from build123d import *

# Parameters (mm, degrees)
SKETCH_1_W          = 75
SKETCH_1_H          = 15
EXTRUDE_1_DEPTH     = 2
FILLET_1_R          = 7.5
SKETCH_2_R          = 4.5
SKETCH_2_R_2        = 2
CUT_EXTRUDE_1_DEPTH = 2
CUT_EXTRUDE_3_DEPTH = 10
FILLET_5_R          = 1


with BuildPart() as part:
    # 草图1 → 凸台-拉伸1 (new body)
    with BuildSketch(Plane.XY):
        Rectangle(SKETCH_1_W, SKETCH_1_H)
    extrude(amount=EXTRUDE_1_DEPTH)

    # 圆角1
    fillet_1_edges = [part.edges().sort_by_distance(p)[0] for p in [
        (37.5, -7.5, 1),
        (-37.5, -7.5, 1),
        (-37.5, 7.5, 1),
        (37.5, 7.5, 1),
    ]]
    fillet(fillet_1_edges, radius=FILLET_1_R - 0.0001)  # a hair under: the kernel refuses the full size

    # 草图2 → 切除-拉伸1 (cut)
    with BuildSketch(Plane.XY.offset(2)):
        with Locations((30, 0)):
            Circle(SKETCH_2_R)
        with Locations((-30, 0)):
            Circle(SKETCH_2_R_2)
    extrude(amount=-CUT_EXTRUDE_1_DEPTH, mode=Mode.SUBTRACT)

    # 草图3 → 切除-拉伸3 (cut)
    with BuildSketch(Plane.XY.offset(2)):
        Polygon((-17.890227771, -5), (0, -1.024393829), (17.890227771, -5), align=None)
        Polygon((-22.5, -3.975606171), (-22.5, 3.975606171), (-4.609772229, 0), align=None)
        Polygon((-17.890227771, 5), (17.890227771, 5), (0, 1.024393829), align=None)
        Polygon((22.5, -3.975606171), (22.5, 3.975606171), (4.609772229, 0), align=None)
    extrude(amount=-CUT_EXTRUDE_3_DEPTH, mode=Mode.SUBTRACT)

    # 圆角5
    fillet_5_edges = [part.edges().sort_by_distance(p)[0] for p in [
        (0, 1.024393829, 1),
        (-17.890227771, 5, 1),
        (17.890227771, 5, 1),
        (4.609772229, 0, 1),
        (22.5, 3.975606171, 1),
        (22.5, -3.975606171, 1),
        (0, -1.024393829, 1),
        (17.890227771, -5, 1),
        (-17.890227771, -5, 1),
        (-22.5, 3.975606171, 1),
        (-4.609772229, 0, 1),
        (-22.5, -3.975606171, 1),
    ]]
    fillet(fillet_5_edges, radius=FILLET_5_R)


solid = part.part
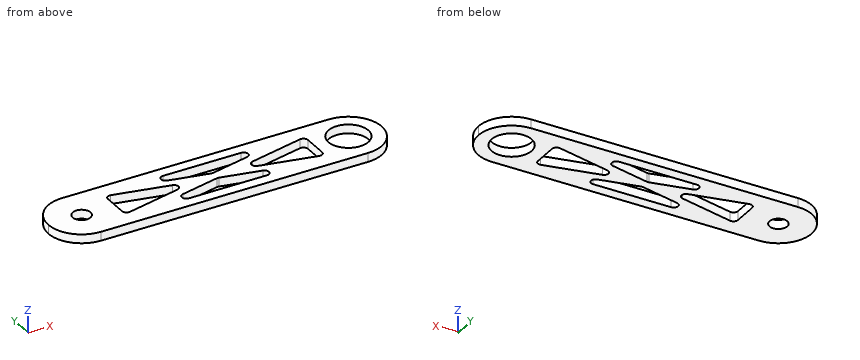
Input: part model. Units: mm. Frame: model coordinates. Coordinates: 2 decimals unless noted, no trailing zeros. Write each loop counter-clockwise with the first axis right and the second up, starting at its lowest first coordinate (ties: lowest second). Pieces come first, ordered by that corner, then holes. Notation, with made-up numbers: M -9.5,83.25 L 23.5,83.25 A25 cw 23.5,119.25 Z; hole C -15,7 d4. An arc over 180 degrees is marked long. Answer as a JSON object with one key per item and string values. Group by question number.
(1) Section B-B on x = -7. Output: boundary loops of the cut face in (y, z).
(2) Ray query, line 1 along Y through (x, z) = (-30, 0.7); line 2 along Y through (x, z) = (30, 1.15); line 3 along X through (y, z) = (4, 1.5). Return the intervals inside material, ascending. Write a range as [from, to].
(3) Section A-A on z = 0.55. Give the number of separate pieces and of enclosed holes in the cut face, plus the area to 3 significant figures.
(4) Contact query for flat-ended pins moving along their axis: P1, Ø1, axis at y = 6, z = 0.5, coming from the +X side; P2, Ø3.5, axis at x = -30, y = 0, coming from the +Z side; P3, Ø1, axis at y = 1, z = 0.5, coming from the -X side. Output: stop coordinate, or through.
(5) Section C-C on x = -14.5. Output: boundary loops of the cut face in (y, z), plus the area to 3 significant figures.
Result set:
{
 "1": {"outline": "M -7.5,0 L -5,0 L -5,2 L -7.5,2 Z; M -2.58,0 L 2.58,0 L 2.58,2 L -2.58,2 Z; M 5,0 L 7.5,0 L 7.5,2 L 5,2 Z"},
 "2": {"line 1": "y = [-7.5, -2], [2, 7.5]", "line 2": "y = [-7.5, -4.5], [4.5, 7.5]", "line 3": "x = [-36.34, -9.78], [9.78, 27.94], [32.06, 36.34]"},
 "3": {"separate pieces": "1", "enclosed holes": "6", "area": "754 mm2"},
 "4": {"P1": "stops at x = 35.1", "P2": "passes through", "P3": "stops at x = -37.48"},
 "5": {"outline": "M -7.5,0 L -2.2,0 L -2.2,2 L -7.5,2 Z; M 2.2,0 L 7.5,0 L 7.5,2 L 2.2,2 Z", "area": "21.2 mm2"}
}
